Geometry check sheet. Reference: the model listing, model coordinates, mm. A direction names the side the tool comes from. Round coordinates to 2 decimals unless told otherwise and drop trailing zeros. Write each loop counter-clockwise with the first axis right and the second up, starting at its lowest first coordinate (ties: lowest second). Pieces come first, ordered by that corner, then holes.
Item 1: Cross-section at C-C (z = 13.5). Enter the section's corners in (x, y).
Item 2: Cross-section at B-B (z = 6.25). Enter the section's corners in (x, y).
Item 3: Cross-section at A-A (x = 0). Enter the section's corners in (y, z).
Item 4: Depth check by flat-ended pin: P1, Ø1, axis at y = 0.5, z = 15.5, coming from the -X side; P2, Ø1, axis at y = 10, z = 16, coming from the +X side; P3, Ø2, axis at y = -6, z = 13, coming from the +X side. Enter the tip coordinate at first touch or a pass-through.
Item 5: Access from +Z, -Z, +X, -X, +Y, -Y to the whole of each face (thin tool, end or side, straight path). Record for faces 4 (the face through (2, 11.9, 18)), 5 (the face through (12, 0, 8.672)), 6 (the face through (-1.17, -12.59, 20.2)), 7 (the face through (-16, 0, 0)), 8 (the face through (9, 0, 6.695)).
Item 6: Draft check along Z on faces 1 (the face through (-12, 0, 8.672)), 2 (the face through (-13.9, 0, 1)), 3 (the face through (-8, 0, 5)). Enter one of: pulls with the +Z half, pulls with the -Z half, needs draft (parallel to the pull), parting line crosses it, or undercut.
Item 7: Scan lines: probe 1 along X at (y, z) = (0.75, 2.75); probe 2 along Z at (x, y) = (0, -12.5); probe 3 along Z at (x, y) = (0, -14.4). Record each from-to range of solid material in increasing order.
from build123d import *

# Parameters (mm, degrees)
F0_R     = 7.65
F1_DEPTH = 14.9
F3_R     = 8.95
F4_DEPTH = 1
F5_R     = 7.65
F5_R_2   = 6.65
F6_DEPTH = 3
F7_R     = 8.45
F8_DEPTH = 2.8


with BuildPart() as f1:
    # F0 (on Front) → F1 (new body, symmetric)
    with BuildSketch(Plane.XZ):
        Polygon((6.1629465781, 0.6753290654), (6.1629465781, 0), (9.6, 0), (9.6, 2.6953140035), (8, 2.6953140035), (8, 6.6953140035), (9.6, 6.6953140035), (9.6, 8.6722822437), (13.9, 8.6722822437), (13.9, 6.6953140035), (15.5, 6.6953140035), (15.5, 2.6953140035), (13.9, 2.6953140035), (13.9, 0), (18.25, 0), (18.25, 8.7399063632), (14.7912298739, 11.2948538736), (11.3324597478, 11.2948538736), (9.5360150372, 18.1063750603), (6.6399620846, 20.6953901798), (0, 20.6953901798), (-6.6399620846, 20.6953901798), (-9.5360150372, 18.1063750603), (-11.3324597478, 11.2948538736), (-14.7912298739, 11.2948538736), (-18.25, 8.7399063632), (-18.25, 0), (-13.9, 0), (-13.9, 2.6953140035), (-15.5, 2.6953140035), (-15.5, 6.6953140035), (-13.9, 6.6953140035), (-13.9, 8.6722822437), (-9.6, 8.6722822437), (-9.6, 6.6953140035), (-8, 6.6953140035), (-8, 2.6953140035), (-9.6, 2.6953140035), (-9.6, 0), (-6.1629465781, 0), (-6.1629465781, 0.6753290654), (0, 0.6753290654), align=None)
        with Locations((0, 11.3253290654)):
            Circle(F0_R, mode=Mode.SUBTRACT)
    extrude(amount=F1_DEPTH, both=True)

    # F3 (on offset) → F4 (cut)
    with BuildSketch(Plane.XZ.offset(12.1)):
        with Locations((0, 11.3253290654)):
            Circle(F3_R)
    extrude(amount=F4_DEPTH, mode=Mode.SUBTRACT)

    # F5 (on face) → F6 (join)
    with BuildSketch(Plane(origin=(0, 14.9, 0), x_dir=(-1, 0, 0), z_dir=(0, 1, 0))):
        with Locations((0, 11.3253290654)):
            Circle(F5_R)
        with Locations((0, 11.3253290654)):
            Circle(F5_R_2, mode=Mode.SUBTRACT)
    extrude(amount=-F6_DEPTH)

    # F7 (on face) → F8 (cut, through all)
    with BuildSketch(Plane.XZ.offset(14.9)):
        with Locations((0, 11.3253290654)):
            Circle(F7_R)
    extrude(amount=-F8_DEPTH, mode=Mode.SUBTRACT)


solid = f1.part
Resolved:
1. outline: (-10.75, -14.9) - (-8.17, -14.9) - (-8.17, -13.1) - (-8.68, -13.1) - (-8.68, -12.1) - (-7.33, -12.1) - (-7.33, 11.9) - (-6.28, 11.9) - (-6.28, 14.9) - (-10.75, 14.9) - close; (6.28, 11.9) - (7.33, 11.9) - (7.33, -12.1) - (8.68, -12.1) - (8.68, -13.1) - (8.17, -13.1) - (8.17, -14.9) - (10.75, -14.9) - (10.75, 14.9) - (6.28, 14.9) - close
2. outline: (-18.25, -14.9) - (-15.5, -14.9) - (-15.5, 14.9) - (-18.25, 14.9) - close; (-8, -14.9) - (-6.76, -14.9) - (-6.76, -13.1) - (-7.37, -13.1) - (-7.37, -12.1) - (-5.72, -12.1) - (-5.72, 11.9) - (-4.3, 11.9) - (-4.3, 14.9) - (-8, 14.9) - close; (4.3, 11.9) - (5.72, 11.9) - (5.72, -12.1) - (7.37, -12.1) - (7.37, -13.1) - (6.76, -13.1) - (6.76, -14.9) - (8, -14.9) - (8, 14.9) - (4.3, 14.9) - close; (15.5, -14.9) - (18.25, -14.9) - (18.25, 14.9) - (15.5, 14.9) - close
3. outline: (-14.9, 0.68) - (14.9, 0.68) - (14.9, 4.68) - (11.9, 4.68) - (11.9, 3.68) - (-12.1, 3.68) - (-12.1, 2.38) - (-13.1, 2.38) - (-13.1, 2.88) - (-14.9, 2.88) - close; (-14.9, 19.78) - (-13.1, 19.78) - (-13.1, 20.28) - (-12.1, 20.28) - (-12.1, 18.98) - (11.9, 18.98) - (11.9, 17.98) - (14.9, 17.98) - (14.9, 20.7) - (-14.9, 20.7) - close
4. P1: stops at x = -10.36
4. P2: stops at x = 10.22
4. P3: stops at x = 11.15
5. face 4: -Y
5. face 5: -Z, +Y, -Y
5. face 6: none
5. face 7: -Z, +X, -X, +Y, -Y
5. face 8: +Y, -Y
6. face 1: pulls with the -Z half
6. face 2: needs draft
6. face 3: undercut
7. probe 1: x = -18.25 to -15.5, -8 to 8, 15.5 to 18.25
7. probe 2: z = 0.68 to 2.38, 20.28 to 20.7
7. probe 3: z = 0.68 to 2.88, 19.78 to 20.7
